Here's how the part is built. I have some questions about the finished solid (model axes, mm). A direction names the side the tool comes from. Give positions to 0.01 mm unless a question says otherwise; leave off trailing zeros. Order: outer loops, then holes, each group sorted by start corner. A loop starts at its lowest first (then second) coordinate and runs counter-clockwise, first axis right, second up.
from build123d import *

# Parameters (mm, degrees)
BOSS_EXTRUDE1_DEPTH = 3
SKETCH4_R           = 5
CUT_EXTRUDE1_DEPTH  = 10.4
SKETCH7_W           = 6.5
SKETCH7_H           = 3
CUT_REVOLVE1_ANGLE  = 90
SKETCH8_R           = 3.25
CUT_EXTRUDE2_DEPTH  = 119.886500495
SKETCH9_W           = 16
SKETCH9_H           = 18
BOSS_EXTRUDE2_DEPTH = 6
SKETCH10_R          = 4
CUT_EXTRUDE3_DEPTH  = 8
FILLET1_R           = 8
FILLET2_R           = 9
SKETCH11_W          = 3
SKETCH11_H          = 15
BOSS_EXTRUDE3_DEPTH = 8
FILLET3_R           = 3
FILLET4_R           = 6
SKETCH12_W          = 40
SKETCH12_H          = 3
SKETCH12_W_2        = 20
BOSS_EXTRUDE4_DEPTH = 1.8
CHAMFER1_SIZE       = 2
CHAMFER1_SIZE_2     = 3.464101615


# Some blends are built 0.0001 mm under size
with BuildPart() as part:
    # Sketch1 → Boss-Extrude1 (new body)
    with BuildSketch(Plane.XY):
        Polygon((-12.5, 0), (-12.5, -70), (-25, -70), (-25, -110), (15, -110), (15, -70), (12.5, -70), (12.5, -25), (45, -25), (45, -10), (12.5, -10), (12.5, 0), (0, 0), align=None)
    extrude(amount=BOSS_EXTRUDE1_DEPTH)

    # Sketch4 → Cut-Extrude1 (cut)
    with BuildSketch(Plane.XY.offset(3)):
        with Locations((0, -100)):
            Circle(SKETCH4_R)
    extrude(amount=-CUT_EXTRUDE1_DEPTH, mode=Mode.SUBTRACT)

    # Sketch7 → Cut-Revolve1 (revolve, cut)
    with BuildSketch(Plane(origin=(0, -100, 0), x_dir=(1, 0, 0), z_dir=(0, 1, 0))):
        with Locations((-16, -1.5)):
            Rectangle(SKETCH7_W, SKETCH7_H)
    revolve(axis=Axis((0, -100, -80.99), (0, 0, -1)), revolution_arc=CUT_REVOLVE1_ANGLE, mode=Mode.SUBTRACT)

    # Sketch8 → Cut-Extrude2 (cut, through all)
    with BuildSketch(Plane.XY):
        with Locations((0, -84)):
            Circle(SKETCH8_R)
        with Locations((-16, -100)):
            Circle(SKETCH8_R)
    extrude(amount=CUT_EXTRUDE2_DEPTH, mode=Mode.SUBTRACT)

    # Sketch9 → Boss-Extrude2 (add)
    with BuildSketch(Plane(origin=(0, 0, 0), x_dir=(0, 0, -1), z_dir=(1, 0, 0))):
        with Locations((-8, 9)):
            Rectangle(SKETCH9_W, SKETCH9_H)
    extrude(amount=-BOSS_EXTRUDE2_DEPTH)

    # Sketch10 → Cut-Extrude3 (cut)
    with BuildSketch(Plane(origin=(0, 0, 0), x_dir=(0, 0, -1), z_dir=(1, 0, 0))):
        with Locations((-8, 9)):
            Circle(SKETCH10_R)
    extrude(amount=-CUT_EXTRUDE3_DEPTH, mode=Mode.SUBTRACT)

    # Fillet1
    fillet1_edges = [part.edges().sort_by_distance(p)[0] for p in [
        (-3, 0, 16),
        (-3, 18, 0),
        (-3, 18, 16),
    ]]
    fillet(fillet1_edges, radius=FILLET1_R - 0.0001)  # a hair under: the kernel refuses the full size

    # Fillet2
    # the kernel refuses this fillet: 9 mm, written as the material it adds along each edge
    with BuildSketch(Plane(origin=(-6, 0, 3), x_dir=(0, 0.032615873538584784, 0.9994679608638364), z_dir=(1, 0, 0))) as fillet2_piece_1:
        with BuildLine():
            CenterArc((8.717235267, 8.811741396), FILLET2_R, 181.869083386, 76.391304548)
            Line((-0.27797638, 8.518198535), (-1.177497545, 8.488844248))
            Line((-1.177497545, 8.488844248), (-0.899521165, -0.029354286))
            Line((-0.899521165, -0.029354286), (0.029354286, -0.899521165))
            ThreePointArc((0.029354286, -0.899521165), (5.026794037, -0.736438535), (6.702939259, -0.88117414))
            Line((6.702939259, -0.88117414), (6.886057078, 0))
        make_face()
    extrude(amount=6)

    # Sketch11 → Boss-Extrude3 (add)
    with BuildSketch(Plane.XY.offset(3)):
        with Locations((43.5, -17.5)):
            Rectangle(SKETCH11_W, SKETCH11_H)
    extrude(amount=BOSS_EXTRUDE3_DEPTH)

    # Fillet3
    fillet3_edges = [part.edges().sort_by_distance(p)[0] for p in [
        (42, -17.5, 3),
        (45, -17.5, 0),
    ]]
    fillet(fillet3_edges, radius=FILLET3_R)

    # Fillet4
    # the kernel refuses this fillet: 6 mm, written as the material it adds along each edge
    with BuildSketch(Plane(origin=(12.5, -25, 0), x_dir=(1, 0, 0), z_dir=(0, 0, 1))) as fillet4_piece_1:
        with BuildLine():
            CenterArc((FILLET4_R, -FILLET4_R), FILLET4_R, 90, 90)
            Line((0, -FILLET4_R), (0, 0))
            Line((0, 0), (FILLET4_R, 0))
        make_face()
    extrude(amount=3)
    with BuildSketch(Plane(origin=(12.5, -70, 0), x_dir=(0, 1, 0), z_dir=(0, 0, 1))) as fillet4_piece_2:
        with BuildLine():
            CenterArc((4.873397172, -6), FILLET4_R, 90, 54.314665287)
            Line((0, -2.5), (0, 0))
            Line((0, 0), (4.873397172, 0))
        make_face()
    extrude(amount=3)
    with BuildSketch(Plane(origin=(-12.5, -70, 0), x_dir=(0, 1, 0), z_dir=(0, 0, 1))) as fillet4_piece_3:
        with BuildLine():
            CenterArc((FILLET4_R, FILLET4_R), FILLET4_R, 180, 90)
            Line((0, FILLET4_R), (0, 0))
            Line((0, 0), (FILLET4_R, 0))
        make_face()
    extrude(amount=3)
    # the kernel refuses this fillet: 6 mm, written as the material it takes off along each edge
    with BuildSketch(Plane(origin=(15, -110, -15), x_dir=(0, 1, 0), z_dir=(0, 0, 1)), Plane(origin=(-25, -110, -15), x_dir=(1, 0, 0), z_dir=(0, 0, 1)), Plane(origin=(-25, -70, -15), x_dir=(0, -1, 0), z_dir=(0, 0, 1))) as fillet4_2_piece_1:
        with BuildLine():
            CenterArc((FILLET4_R, FILLET4_R), FILLET4_R, 180, 90)
            Line((0, FILLET4_R), (0, 0))
            Line((0, 0), (FILLET4_R, 0))
        make_face()
    extrude(amount=33, mode=Mode.SUBTRACT)
    with BuildSketch(Plane(origin=(-12.5, 0, -15), x_dir=(1, 0, 0), z_dir=(0, 0, 1)), Plane(origin=(12.5, 0, -15), x_dir=(0, -1, 0), z_dir=(0, 0, 1))) as fillet4_2_piece_2:
        with BuildLine():
            CenterArc((FILLET4_R, -FILLET4_R), FILLET4_R, 90, 90)
            Line((0, -FILLET4_R), (0, 0))
            Line((0, 0), (FILLET4_R, 0))
        make_face()
    extrude(amount=33, mode=Mode.SUBTRACT)

    # Sketch12 → Boss-Extrude4 (add)
    with BuildSketch(Plane.XY.offset(3)):
        with Locations((10, -17.5)):
            Rectangle(SKETCH12_W, SKETCH12_H)
        with Locations((0, -43.5)):
            Rectangle(SKETCH12_W_2, SKETCH12_H)
    extrude(amount=BOSS_EXTRUDE4_DEPTH)

    # Chamfer1
    # the kernel refuses this chamfer: 3.464101615, 2 mm, written as the material it takes off along each edge
    with BuildSketch(Plane(origin=(10, -53.961927941, 4.8), x_dir=(0, 0, -1), z_dir=(0, 1, 0))) as chamfer1_piece_1_section:
        Polygon((CHAMFER1_SIZE, 0), (0, CHAMFER1_SIZE_2), (0, 0), align=None)
    chamfer1_piece_1 = extrude(amount=20.923855882, mode=Mode.PRIVATE)
    chamfer1_piece_1 = split(chamfer1_piece_1, bisect_by=Plane(origin=(10, -53.961927941, 3), z_dir=(0, 0, 1)), keep=Keep.TOP, mode=Mode.PRIVATE)
    add(chamfer1_piece_1, mode=Mode.SUBTRACT)
    with BuildSketch(Plane(origin=(-10, -33.038072059, 4.8), x_dir=(0, 0, -1), z_dir=(0, -1, 0))) as chamfer1_piece_2_section:
        Polygon((CHAMFER1_SIZE, 0), (0, CHAMFER1_SIZE_2), (0, 0), align=None)
    chamfer1_piece_2 = extrude(amount=20.923855882, mode=Mode.PRIVATE)
    chamfer1_piece_2 = split(chamfer1_piece_2, bisect_by=Plane(origin=(-10, -33.038072059, 3), z_dir=(0, 0, 1)), keep=Keep.TOP, mode=Mode.PRIVATE)
    add(chamfer1_piece_2, mode=Mode.SUBTRACT)
    with BuildSketch(Plane(origin=(-10, -7.038072059, 4.8), x_dir=(0, 0, -1), z_dir=(0, -1, 0))) as chamfer1_piece_3_section:
        Polygon((CHAMFER1_SIZE, 0), (0, CHAMFER1_SIZE_2), (0, 0), align=None)
    chamfer1_piece_3 = extrude(amount=20.923855882, mode=Mode.PRIVATE)
    chamfer1_piece_3 = split(chamfer1_piece_3, bisect_by=Plane(origin=(-10, -7.038072059, 3), z_dir=(0, 0, 1)), keep=Keep.TOP, mode=Mode.PRIVATE)
    add(chamfer1_piece_3, mode=Mode.SUBTRACT)
    with BuildSketch(Plane(origin=(30, -27.961927941, 4.8), x_dir=(0, 0, -1), z_dir=(0, 1, 0))) as chamfer1_piece_4_section:
        Polygon((CHAMFER1_SIZE, 0), (0, CHAMFER1_SIZE_2), (0, 0), align=None)
    chamfer1_piece_4 = extrude(amount=20.923855882, mode=Mode.PRIVATE)
    chamfer1_piece_4 = split(chamfer1_piece_4, bisect_by=Plane(origin=(30, -27.961927941, 3), z_dir=(0, 0, 1)), keep=Keep.TOP, mode=Mode.PRIVATE)
    add(chamfer1_piece_4, mode=Mode.SUBTRACT)


solid = part.part
Q1. If we section it at A-A on x = -2: Give the number of separate pieces and of enclosed holes in the cut face, plus the area to 3 significant figures.
Filled sheet:
separate pieces: 3
enclosed holes: 1
area: 504 mm2
Q2. If we section it at B-B on y = -84: List the corners of the cut face in (x, z) for me.
Filled sheet:
outline: (-25, 0) - (-10.7, 0) - (-10.7, 3) - (-25, 3) - close; (3.25, 0) - (15, 0) - (15, 3) - (3.25, 3) - close
Q3. If we section it at C-C on y = -17.5: List the corners of the cut face in (x, z) for me.
Filled sheet:
outline: (-12.5, 0) - (42, 0) arc R3 ccw to (45, 3) - (45, 11) - (42, 11) - (42, 6) arc R3 cw to (39, 3) - (29.65, 3) - (26.54, 4.8) - (-6.54, 4.8) - (-9.65, 3) - (-12.5, 3) - close
Q4. I need wall thicknesses on L1, parallel to X at y = 2, z = 6.5; L2, parallel to X at y = -102, z = 1; L3, parallel to Y at x = -1.6, z = 8. Which ranges of each line are inside material? Lowest first, please.
Filled sheet:
L1: x = -6 to 0
L2: x = -25 to -18.56, -13.44 to -4.58, 4.58 to 15
L3: y = -0.46 to 5, 13 to 18
Q5. I'm going to push flat-ended pins straight in: P1, Ø0.9, axis at x = 3, z = 4, coming from the -Y side; P2, Ø1.5, axis at x = -1, y = -80, coming from the +Z side; P3, Ø1.5, axis at y = -45, z = 1, coming from the +X side. Where does each tip first touch, or does it pass through?
Filled sheet:
P1: stops at y = -45
P2: stops at z = 3
P3: stops at x = 12.5
Q6. For faces 4 (the face through (-3.04, -3.02, 4.88)), 5 (the face through (0, -43, 4.8)), 6 (the face through (12.5, -48, 1)), 7 (the face through (12.5, -8, 1)), 8 (the face through (-9.11, -91.08, 1.48)), which set-ups out of +Z, -Z, +X, -X, +Y, -Y let a thin tool reach every point of the face, with its end or its side?
Filled sheet:
face 4: +Z, +X, -X
face 5: +Z, +X, -X, -Y
face 6: +Z, -Z, +X
face 7: +Z, -Z, +X, +Y
face 8: +Z, -Z
Q7. If we section it at D-D on x = -16: List the corners of the cut face in (y, z) for me, plus the area to 3 significant figures.
Filled sheet:
outline: (-110, 0) - (-103.25, 0) - (-103.25, 3) - (-110, 3) - close; (-89.3, 0) - (-69.45, 0) - (-69.45, 3) - (-89.3, 3) - close
area: 79.8 mm2
Q8. Thinking about a two-plate mould opening in X: for faces 1 (the face through (14.304, -26.711, 1.479)), 2 (the face through (3.25, -84.07, 1.48)), 3 (the face through (-10.696, -1.711, 1.479)), which applies, released by +X, released by -X, zero draft, split by the parting line, or undercut?
Filled sheet:
face 1: released by +X
face 2: undercut
face 3: released by -X
